from build123d import *

# Parameters (mm, degrees)
F1_DEPTH = 2


with BuildPart() as f1:
    # F0 (on Front) → F1 (new body)
    with BuildSketch(Plane.XZ):
        with BuildLine():
            ThreePointArc((13.1280048062, -7.2564102564), (14.5244633652, -3.746993989), (15, 0))
            ThreePointArc((15, 0), (14.5244633652, 3.746993989), (13.1280048062, 7.2564102564))
            ThreePointArc((13.1280048062, 7.2564102564), (0, 1.548676929), (-13.1280048062, 7.2564102564))
            ThreePointArc((-13.1280048062, 7.2564102564), (-15, 0), (-13.1280048062, -7.2564102564))
            ThreePointArc((-13.1280048062, -7.2564102564), (0, -1.548676929), (13.1280048062, -7.2564102564))
        make_face()
        with BuildLine():
            ThreePointArc((-13.1280048062, 7.2564102564), (0, 1.548676929), (13.1280048062, 7.2564102564))
            ThreePointArc((13.1280048062, 7.2564102564), (0, 15), (-13.1280048062, 7.2564102564))
        make_face()
        with BuildLine():
            ThreePointArc((-13.1280048062, 7.2564102564), (0, 15), (13.1280048062, 7.2564102564))
            ThreePointArc((13.1280048062, 7.2564102564), (15.8589994188, 11.0891654734), (17.5, 15.5))
            Line((17.5, 15.5), (17.5, 19.5))
            Line((17.5, 19.5), (10.5, 19.5))
            Line((10.5, 19.5), (10.5, 17.5))
            Line((10.5, 17.5), (-10.5, 17.5))
            Line((-10.5, 17.5), (-10.5, 19.5))
            Line((-10.5, 19.5), (-17.5, 19.5))
            Line((-17.5, 19.5), (-17.5, 15.5))
            ThreePointArc((-17.5, 15.5), (-15.8589994188, 11.0891654734), (-13.1280048062, 7.2564102564))
        make_face()
        with BuildLine():
            ThreePointArc((17.5, -15.5), (15.8589994188, -11.0891654734), (13.1280048062, -7.2564102564))
            ThreePointArc((13.1280048062, -7.2564102564), (0, -15), (-13.1280048062, -7.2564102564))
            ThreePointArc((-13.1280048062, -7.2564102564), (-15.8589994188, -11.0891654734), (-17.5, -15.5))
            Line((-17.5, -15.5), (-17.5, -19.5))
            Line((-17.5, -19.5), (-10.5, -19.5))
            Line((-10.5, -19.5), (-10.5, -17.5))
            Line((-10.5, -17.5), (10.5, -17.5))
            Line((10.5, -17.5), (10.5, -19.5))
            Line((10.5, -19.5), (17.5, -19.5))
            Line((17.5, -19.5), (17.5, -15.5))
        make_face()
        with BuildLine():
            ThreePointArc((-13.1280048062, -7.2564102564), (0, -15), (13.1280048062, -7.2564102564))
            ThreePointArc((13.1280048062, -7.2564102564), (0, -1.548676929), (-13.1280048062, -7.2564102564))
        make_face()
    extrude(amount=F1_DEPTH)


solid = f1.part
Verification items for the finished model (mm, model axes). A direction names the side the tool comes from. Give positions to 0.01 mm unless a question says otherwise; leave off trailing zeros. Loops run counter-clockwise (first coordinate to the right, second up) from the corner with the lowest first, then second, coordinate; pieces in that order, holes last. Notation, with made-up numbers: (-19.5, -24.75) - (24.5, -24.75) arc R22 cw to (24.5, 5.25) - close; hole circle Ø7 at (87.25, -12.5). An arc over 180 degrees is marked (long way). Write item = value, one per line. Start each with the question number.
Q1. Depth check by flat-ended pin: P1, Ø1, axis at x = -5, y = -0.5, coming from the -Z side. Enter the tip coordinate at first touch or a pass-through.
Q2. Cross-section at B-B, the plane y = -1.6. Enter the section's corners in (x, z).
Q3. Tool access check on faces 1 (the face through (0, -1, -17.5)), 2 (the face through (10.5, -1, 19)), 3 (the face through (-15.89, -0.99, 11.15)), 4 (the face through (0, 0, 0)), 5 (the face through (15.828, -0.986, 11.031)). Record the directions out of +Z, -Z, +X, -X, +Y, -Y that give a thin tool (end or side, any length) a straight path to the whole face; none if there is none.
Q4. Cross-section at A-A, the plane x = 14. Enter the section's corners in (y, z).
Q5. Mould release check, pull along X, two halves, no side actions. Record for faces 6 (the face through (-14, -1, 19.5)), 7 (the face through (-15.828, -0.986, -11.031)), 8 (the face through (-10.5, -1, 18)): released by +X, released by -X, zero draft, split by the parting line, or undercut.
Q6. Cross-section at C-C, the plane z = 5. Enter the section's corners in (x, y), and give its area (3 significant figures).
Q7. Thickness scan on line 1 (X direction, y = -0.6, z = 18); line 2 (Z direction, x = 1.5, y = -0.2); line 3 (X direction, y = -1, z = 9.5). Record the ranges inside material, lowest first.
Q8. Cross-section at D-D, the plane x = 7. Enter the section's corners in (y, z), and give its area (3 significant figures).
Answer key:
q1.P1 = -17.5
q2.outline = (-17.5, -19.5) - (-10.5, -19.5) - (-10.5, -17.5) - (10.5, -17.5) - (10.5, -19.5) - (17.5, -19.5) - (17.5, -15.5) arc R17.95 ccw to (13.13, -7.26) arc R15 ccw to (13.13, 7.26) arc R17.95 ccw to (17.5, 15.5) - (17.5, 19.5) - (10.5, 19.5) - (10.5, 17.5) - (-10.5, 17.5) - (-10.5, 19.5) - (-17.5, 19.5) - (-17.5, 15.5) arc R17.95 ccw to (-13.13, 7.26) arc R15 ccw to (-13.13, -7.26) arc R17.95 ccw to (-17.5, -15.5) - close
q3.face_1 = -Z, +Y, -Y
q3.face_2 = +Z, +Y, -Y
q3.face_3 = -X, +Y, -Y
q3.face_4 = +Z, -Z, +X, -X, +Y
q3.face_5 = +X, +Y, -Y
q4.outline = (-2, -19.5) - (0, -19.5) - (0, -8.26) - (-2, -8.26) - close; (-2, -5.39) - (0, -5.39) - (0, 5.39) - (-2, 5.39) - close; (-2, 8.26) - (0, 8.26) - (0, 19.5) - (-2, 19.5) - close
q5.face_6 = zero draft
q5.face_7 = released by -X
q5.face_8 = undercut
q6.outline = (-14.14, -2) - (14.14, -2) - (14.14, 0) - (-14.14, 0) - close
q6.area = 56.6 mm^2
q7.line_1 = -17.5 to -10.5, 10.5 to 17.5
q7.line_2 = -17.5 to 17.5
q7.line_3 = -14.91 to 14.91
q8.outline = (-2, -17.5) - (0, -17.5) - (0, 17.5) - (-2, 17.5) - close
q8.area = 70.0 mm^2
